Geometry check sheet. Reference: the model listing, model coordinates, mm. Round coordinates to 2 decimals unless told otherwise and drop trailing zeros. Order: outer loops, then holes, each group sorted by start corner. A loop starts at its lowest first (then second) coordinate and runs counter-clockwise, first axis right, second up.
```python
from build123d import *

# Parameters (mm, degrees)
BOSS_EXTRUDE1_DEPTH = 381
CUT_EXTRUDE1_REACH  = 383.687
SKETCH2_R           = 3.175
SKETCH3_R           = 2.54
CUT_EXTRUDE2_DEPTH  = 7.62
CUT_EXTRUDE3_START  = -7.62
SKETCH4_R           = 2.54
CUT_EXTRUDE3_DEPTH  = 7.62
SKETCH5_W           = 6.35
SKETCH5_H           = 6.35
CUT_EXTRUDE4_DEPTH  = 345.44


with BuildPart() as part:
    # Sketch1 → Boss-Extrude1 (new body)
    with BuildSketch(Plane.XY):
        Polygon((0, 0), (-12.7, 0), (-12.7, 19.05), (-6.35, 19.05), (-6.35, 6.35), (0, 6.35), align=None)
    extrude(amount=-BOSS_EXTRUDE1_DEPTH)

    # Sketch2 → Cut-Extrude1 (cut, up to next)
    with BuildSketch(Plane.ZY.offset(12.7), mode=Mode.PRIVATE) as cut_extrude1_sk1:
        with Locations(Location((-365.76, 12.065, 0), (0, 0, 270))):
            Circle(SKETCH2_R)
    cut_extrude1_tool1 = extrude(cut_extrude1_sk1.sketch, amount=-CUT_EXTRUDE1_REACH, mode=Mode.PRIVATE) & part.part
    add(cut_extrude1_tool1.solids().sort_by_distance((-12.7, 12.065, -365.76))[0], mode=Mode.SUBTRACT)

    # Sketch3 → Cut-Extrude2 (cut)
    with BuildSketch(Plane(origin=(0, 19.05, 0), x_dir=(1, 0, 0), z_dir=(0, 1, 0))):
        with Locations(Location((-9.525, 6.35, 0), (0, 0, 270))):
            Circle(SKETCH3_R)
        with Locations(Location((-9.525, 374.65, 0), (0, 0, 270))):
            Circle(SKETCH3_R)
    extrude(amount=-CUT_EXTRUDE2_DEPTH, mode=Mode.SUBTRACT)

    # Sketch4 → Cut-Extrude3 (cut)
    with BuildSketch(Plane.XZ.offset(CUT_EXTRUDE3_START)):
        with Locations(Location((-9.525, -374.65, 0), (0, 0, 90))):
            Circle(SKETCH4_R)
        with Locations(Location((-9.525, -6.35, 0), (0, 0, 90))):
            Circle(SKETCH4_R)
    extrude(amount=CUT_EXTRUDE3_DEPTH, mode=Mode.SUBTRACT)

    # Sketch5 → Cut-Extrude4 (cut)
    with BuildSketch(Plane(origin=(0, 0, -381), x_dir=(-1, 0, 0), z_dir=(0, 0, -1))):
        with Locations((3.175, 3.175)):
            Rectangle(SKETCH5_W, SKETCH5_H)
    extrude(amount=-CUT_EXTRUDE4_DEPTH, mode=Mode.SUBTRACT)


solid = part.part
```
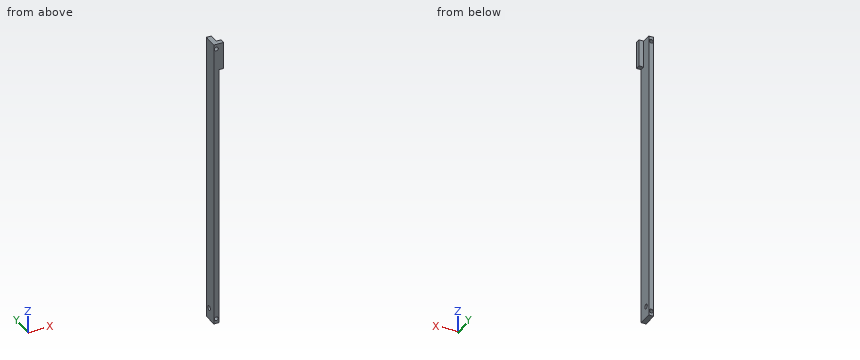
(1) Sectioned sample at B-B, the plane x = -4. Record the cut outline in (y, z).
Returned:
outline: (0, -35.56) - (6.35, -35.56) - (6.35, 0) - (0, 0) - close
(2) Sectioned sample at C-C, the plane z = -325. Record the cut outline in (x, y), and give its area (3 significant figures).
Returned:
outline: (-12.7, 0) - (-6.35, 0) - (-6.35, 19.05) - (-12.7, 19.05) - close
area: 121 mm2
(3) Depth check by flat-ended pin: P1, Ø8.5, axis at y = 12.065, z = -365.76, coming from the -X side; P2, Ø9.5, axis at y = 5.5, z = -236.5, coming from the +X side; P3, Ø3, axis at x = -3, y = 4, coming from the -Z side; P4, Ø3, axis at x = -9.525, z = -374.65, coming from the +Y side. Enter the tip coordinate at first touch or a pass-through.
Returned:
P1: stops at x = -12.7
P2: stops at x = -6.35
P3: stops at z = -35.56
P4: stops at y = 11.43
(4) Sectioned sample at A-A, the plane z = -365.76. Record the cut outline in (x, y).
Returned:
outline: (-12.7, 0) - (-6.35, 0) - (-6.35, 8.89) - (-12.7, 8.89) - close; (-12.7, 15.24) - (-6.35, 15.24) - (-6.35, 19.05) - (-12.7, 19.05) - close
(5) Material ranges on line 1 (X direction, y = 5.5, z = -374.65) (3 decimals); line 2 (X direction, y = 2, z = -6.35) (3 decimals); line 3 (Y direction, x = -10.5, z = -365.76), recorded low to high.
Returned:
line 1: x = -12.7 to -12.065, -6.985 to -6.35
line 2: x = -12.7 to -12.065, -6.985 to 0
line 3: y = 0 to 8.89, 15.24 to 19.05
